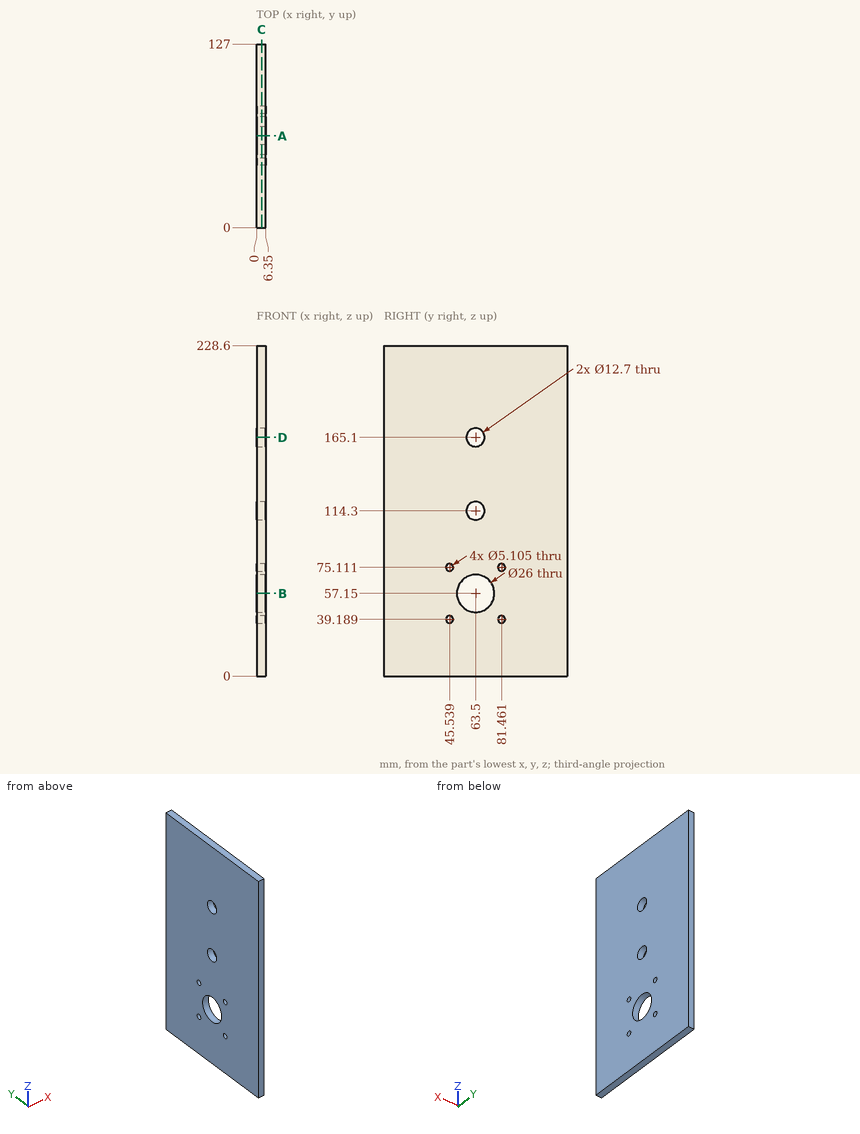
The figure shows three views and two pictorial views of one solid part (mm, origin at its lowest corner). Answer the questions. Give positions to 0.01 mm unless a question says otherwise; leave off trailing zeros. Loops run counter-clockwise (first coordinate to the right, second up) from the corner with the lowest first, then second, coordinate; pieces in that order, holes last. Notation, with made-up numbers: (-18, 30.25) -> (37, 30.25) arc R7 ccw to (37, 35.25) -> close; hole circle Ø7 at (-13, -32.75). An arc over 180 degrees is marked (long way). Use a Markdown table: item, result. Add a question column.
1. A flat-ended cylindrical pin translates along its axis: pin 1 Ø15.5 at (y, z) = (63.5, 57.15) entering from +X. Find the tip coordinate at first contact, or state that the pin passes through.
2. Find the intervals of material crossed by probe 1 along Z at (x, y) = (1.5, 63); probe 2 along Y at (x, z) = (2, 114.3); probe 3 along Z at (x, y) = (5.75, 47) (1 decimal), in increasing order.
3. Section A-A on y = 63.5 is taken. Determine the outline of the cut face in (x, z).
4. Section B-B on z = 57.15 is taken. Determine the outline of the cut face in (x, y).
5. Section D-D on z = 165.1 is taken. Determine the outline of the cut face in (x, y), and give its area (3 significant figures).
6. Section C-C on x = 3.5 is taken. State how many separate pieces and enclosed holes the cut face has, and give its area (3 significant figures).
Results below:
| question | item | result |
|---|---|---|
| 1 | pin 1 | passes through |
| 2 | probe 1 | z = 0 to 44.16, 70.14 to 107.97, 120.63 to 158.77, 171.43 to 228.6 |
| 2 | probe 2 | y = 0 to 57.15, 69.85 to 127 |
| 2 | probe 3 | z = 0 to 37.1, 41.3 to 73, 77.2 to 228.6 |
| 3 | outline | (0, 0) -> (6.35, 0) -> (6.35, 44.15) -> (0, 44.15) -> close; (0, 70.15) -> (6.35, 70.15) -> (6.35, 107.95) -> (0, 107.95) -> close; (0, 120.65) -> (6.35, 120.65) -> (6.35, 158.75) -> (0, 158.75) -> close; (0, 171.45) -> (6.35, 171.45) -> (6.35, 228.6) -> (0, 228.6) -> close |
| 4 | outline | (0, 0) -> (6.35, 0) -> (6.35, 50.5) -> (0, 50.5) -> close; (0, 76.5) -> (6.35, 76.5) -> (6.35, 127) -> (0, 127) -> close |
| 5 | outline | (0, 0) -> (6.35, 0) -> (6.35, 57.15) -> (0, 57.15) -> close; (0, 69.85) -> (6.35, 69.85) -> (6.35, 127) -> (0, 127) -> close |
| 5 | area | 726 mm^2 |
| 6 | separate pieces | 1 |
| 6 | enclosed holes | 7 |
| 6 | area | 28,200 mm^2 |
